The figure shows three views and two pictorial views of one solid part (mm, origin at its lowest corner). Answer the questions. A direction names the side the tool comes from. Coordinates: 2 decimals unless noted, no trailing zeros. Loops run counter-clockwise (first coordinate to the right, second up) from the corner with the lowest first, then second, coordinate; pieces in that order, holes last. Notation, with made-up numbers: M 85.5,15.25 L 112.5,15.25 A23 cw 112.5,27.25 Z; hole C -9.5,44.5 d10. An arc over 180 degrees is marked long. Write each question's results on one line, items separated by ' | '.
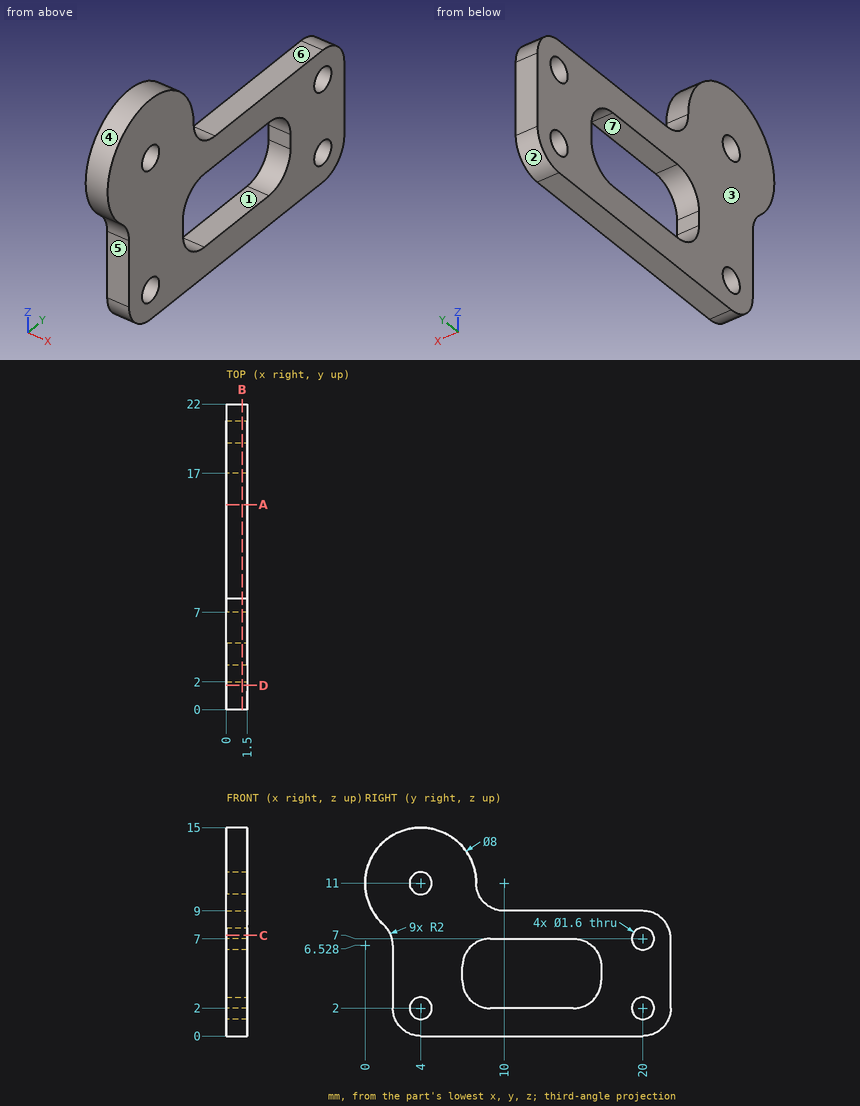
1) Find section A-A, the plane y = 14.75. Give the vertices of the cut face in (x, z), and give its area (3 significant figures).
Check result:
outline: M 0,0 L 1.5,0 L 1.5,2 L 0,2 Z; M 0,7 L 1.5,7 L 1.5,9 L 0,9 Z | area: 6.00 mm^2
2) Find section C-C, the plane z = 7.25. Give the vertices of the cut face in (x, y) (1 decimal).
Check result:
outline: M 0,1.9 L 1.5,1.9 L 1.5,19.2 L 0,19.2 Z; M 0,20.8 L 1.5,20.8 L 1.5,22 L 0,22 Z
3) For a pull along Z with two mould halves and no side action, classify the marked faces 1, 2, 3 and 4 as released by +Z, released by -Z, zero draft, split by the parting line, or undercut.
Check result:
face 1: undercut | face 2: released by -Z | face 3: zero draft | face 4: split by the parting line
4) Straight lines are drawn through the part: probe 1 along Z at (x, y) = (0.75, 15); probe 2 along Y at (x, z) = (0.45, 6.75); probe 3 along Z at (x, y) = (0.3, 16.75). For each, find the intervals that lie inside material, in ascending order. Write a range as [from, to].
Check result:
probe 1: [0, 2], [7, 9] | probe 2: [1.99, 8.03], [15.97, 19.24], [20.76, 22] | probe 3: [0, 3.03], [5.97, 9]
5) Given pin 1 Ø1 at (y, z) = (20, 2) entering from +X; pin 2 Ø8 at (y, z) = (19.5, 5) entering from -X; pin 3 Ø0.8 at (x, z) = (1, 4.5) entering from -Y, each flat-ended and moving along its own axis, determine where each tip first touches the part or whether it passes through.
Check result:
pin 1: through | pin 2: x = 0 | pin 3: y = 2
6) Find section D-D, the plane y = 1.75. Give the vertices of the cut face in (x, z).
Check result:
outline: M 0,7.5 L 1.5,7.5 L 1.5,14.31 L 0,14.31 Z
7) Which of the six approach directions +Z, -Z, +X, -X, +Y, -Y give full straight-line access (tool end or side, diameter ignored) to the marked faces 5, 6 and 7?
Check result:
face 5: -Z, +X, -X, -Y | face 6: +Z, +X, -X, +Y | face 7: +X, -X
8) Find section B-B, the plane x = 1.15. Give the vertices of the cut face in (y, z).
Check result:
outline: M 1.33,8.02 A2 cw 2,6.53 L 2,2 A2 ccw 4,0 L 20,0 A2 ccw 22,2 L 22,7 A2 ccw 20,9 L 10,9 A2 cw 8,11 A4 ccw long Z; hole C 4,2 d1.6; hole C 4,11 d1.6; hole M 7,4 A2 ccw 9,2 L 15,2 A2 ccw 17,4 L 17,5 A2 ccw 15,7 L 9,7 A2 ccw 7,5 Z; hole C 20,2 d1.6; hole C 20,7 d1.6
